For this review, take the finished solid that the model builds, in its own axes (mm). Face numbers are marked on the shaded views. A direction names the side the tool comes from. Give positions to 0.01 mm unless a question says otherwise; leave off trailing zeros. Order: outer loops, then holes, each group sorted by start corner. A loop starts at its lowest first (then second) coordinate and runs counter-clockwise, first axis right, second up.
from build123d import *

# Parameters (mm, degrees)
F0_W     = 26
F0_H     = 3
F1_DEPTH = 24
F0_H_2   = 2.5
F2_DEPTH = 3


with BuildPart() as f1:
    # F0 (on Top) → F1 (new body)
    with BuildSketch(Plane.XY):
        with Locations((0, 11.5)):
            Rectangle(F0_W, F0_H)
        with Locations((0, 6)):
            Rectangle(F0_W, F0_H)
    extrude(amount=F1_DEPTH)

    # F0 (on Top) → F2 (join)
    with BuildSketch(Plane.XY):
        with Locations((0, 11.5)):
            Rectangle(F0_W, F0_H)
        with Locations((0, 8.75)):
            Rectangle(F0_W, F0_H_2)
        with Locations((0, 6)):
            Rectangle(F0_W, F0_H)
        Polygon((0, -13), (13, -13), (13, 4.5), (-13, 4.5), (-13, -13), align=None)
        with BuildLine():
            ThreePointArc((2.5, -4.75), (1.767767, -6.517767), (0, -7.25))
            ThreePointArc((0, -7.25), (-1.767767, -2.982233), (2.5, -4.75))
        make_face(mode=Mode.SUBTRACT)
    extrude(amount=F2_DEPTH)


solid = f1.part
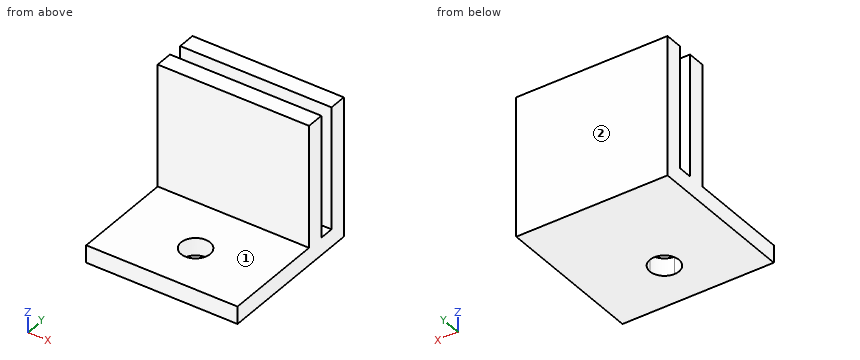
1) Clearance check with flat-ended pins moving along their axes: pin 1 (10.5 mm diameter, centred on x = -0.5, z = 17.5, fed in from -Y); pin 2 (4.5 mm diameter, centred on x = 0, y = -4.75, fed in from +Z). State where each tip first meets the part, or that it passes through.
Answer sheet:
pin 1: stops at y = 4.5
pin 2: passes through
2) We need section C-C on x = 1. Give the boundary of the cut face in (y, z).
Answer sheet:
outline: (-13, 0) - (-7.04, 0) - (-7.04, 3) - (-13, 3) - close; (-2.46, 0) - (13, 0) - (13, 24) - (10, 24) - (10, 3) - (7.5, 3) - (7.5, 24) - (4.5, 24) - (4.5, 3) - (-2.46, 3) - close
3) We need section A-A on x = -7.5. Give the boundary of the cut face in (y, z), then the cut area to 3 significant figures.
Answer sheet:
outline: (-13, 0) - (13, 0) - (13, 24) - (10, 24) - (10, 3) - (7.5, 3) - (7.5, 24) - (4.5, 24) - (4.5, 3) - (-13, 3) - close
area: 204 mm2
4) We need section D-D on y = -10.75. Give the boundary of the cut face in (x, z).
Answer sheet:
outline: (-13, 0) - (13, 0) - (13, 3) - (-13, 3) - close
5) Tool access review of the marked faces 1 and 2: name each direction out of +Z, -Z, +X, -X, +Y, -Y from which nothing blocks a thin tool from reaching the whole face with its end or side.
Answer sheet:
face 1: +Z, +X, -X, -Y
face 2: +Z, -Z, +X, -X, +Y
6) To check wall thickness, follow line 1 (X direction, y = -4.75, z = 2.1); line 2 (Y direction, x = 2.5, z = 5.5); line 3 (Y direction, x = 0, z = 0.7). State the ranges of each line that lie inside material, in increasing order.
Answer sheet:
line 1: x = -13 to -2.5, 2.5 to 13
line 2: y = 4.5 to 7.5, 10 to 13
line 3: y = -13 to -7.25, -2.25 to 13
7) We need section B-B on z = 9.25. Give the boundary of the cut face in (x, y).
Answer sheet:
outline: (-13, 4.5) - (13, 4.5) - (13, 7.5) - (-13, 7.5) - close; (-13, 10) - (13, 10) - (13, 13) - (-13, 13) - close
